Autodesk Inventor part; units mm, degrees
ref_plane "Work Plane2" through (1.7064, 6, 5.9284) normal (0, 0, -1) x (-1, 0, 0)
ref_plane "YZ Plane" through (0, 0, 0) normal (1, 0, 0) x (0, 1, 0)
ref_plane "XZ Plane" through (0, 0, 0) normal (0, 1, 0) x (-1, 0, 0)
sketch "Sketch7" plane through (0, 0, 0) normal (0, 1, 0) x (-1, 0, 0)
  line L0 (-3.4641, -6) -> (-6.9282, 0)
  line L1 (-6.9282, 0) -> (-3.4641, 6)
  line L2 (-3.4641, 6) -> (3.4641, 6)
  line L3 (3.4641, 6) -> (6.9282, 0)
  line L4 (6.9282, 0) -> (3.4641, -6)
  line L5 (3.4641, -6) -> (-3.4641, -6)
  point P0 (0, 0)
  point P1 (0, 0)
  point P2 (0, -6)
  dimension "d24" = 12
extrude "Extrusion6" add sketch "Sketch7" along normal blind 6
sketch "Sketch8" plane through (0, 6, 0) normal (0, 1, 0) x (1, 0, 0)
  circle A0 centre (0, 0) radius 5.5
  circle A1 centre (0, 0) radius 2.575
  line L0 (-0.1332, 2.5716) -> (-0.1332, -1.9284)
  line L1 (-0.1332, -1.9284) -> (-1.7064, -1.9284)
  line L2 (-0.1332, -1.9284) -> (1.7064, -1.9284)
  dimension "d27" = 11
  dimension "d28" = 5.15
  dimension "d29" = 4.5
  dimension "d30" = 1.5732
extrude "Extrusion7" add sketch "Sketch8" along normal blind 18 contours A0 | A1 L1 L2
sketch "Sketch9" plane through (0, 0, 0) normal (0, 0, 1) x (1, 0, 0)
  line L0 (6.9282, 0) -> (3.4641, 0)
  line L1 (6.9282, 0) -> (6.4282, 0)
  line L2 (6.8032, 0.3147) -> (6.4282, 0)
  line L3 (6.9282, 0) -> (6.9282, 0.3868)
  line L4 (0, -4.8) -> (0, 28.8)
  line L5 (6.8032, 0.3147) -> (6.9282, 0.4195)
  line L6 (6.9282, 0.4195) -> (6.9282, 0.3868)
  point P0 (0, 0)
  dimension "d33" = 0.5
  dimension "d35" = 40
  dimension "d39" = 0.125
  dimension "d40" = 0.1049
revolve "Revolution1" cut sketch "Sketch9" angle 360 about axis through (0, -10, 0) along (0, 1, 0)
chamfer "Chamfer3" distance 1 angle 45 2 edges at (0, 24, -2.575) (0, 24, 1.9284)
sketch "Sketch10" plane through (0, 0, 0) normal (0, -1, 0) x (1, 0, 0)
  circle A0 centre (0, 0) radius 1.8
  dimension "d44" = 3.6
extrude "Extrusion8" cut sketch "Sketch10" against normal through all
sketch "Sketch13" plane through (1.7064, 6, 1.9284) normal (0, 0, -1) x (-1, 0, 0)
  circle A0 centre (1.7064, 12) radius 1.8
  point P0 (1.7064, -6)
  dimension "d55" = 3.6
  dimension "d56" = 18
  dimension "d57" = 0
extrude "Extrusion11" cut sketch "Sketch13" against normal through all
ref_plane "Work Plane2" through (1.7064, 6, 5.9284) normal (0, 0, -1) x (-1, 0, 0)
sketch "Sketch14" plane through (1.7064, 6, 5.9284) normal (0, 0, -1) x (-1, 0, 0)
  spline S0 degree 8 poles (3.5064, 12) (3.5064, 12.1901) (3.4834, 12.3798) (3.4377, 12.5672) (3.3691, 12.7503) (3.2769, 12.9271) (3.1607, 13.0947) (3.0198, 13.2496) (2.7182, 13.499) (2.5613, 13.6034) (2.3851, 13.6923) (2.1931, 13.7603) (1.99, 13.8033) (1.7813, 13.819) (1.5725, 13.8069) (1.1492, 13.7262) (0.9448, 13.6548) (0.7585, 13.5594) (0.5918, 13.4445) (0.4454, 13.3144) (0.3197, 13.1725) (0.2144, 13.0225) (0.0308, 12.6885) (-0.0422, 12.5008) (-0.0906, 12.3073) (-0.1146, 12.1105) (-0.1143, 11.9127) (-0.0899, 11.7163) (-0.041, 11.5236) (0.0949, 11.1805) (0.1748, 11.0279) (0.2727, 10.8814) (0.3891, 10.7428) (0.5244, 10.6146) (0.6789, 10.4998) (0.8523, 10.4022) (1.2226, 10.2556) (1.417, 10.2039) (1.6217, 10.1768) (1.8302, 10.1772) (2.0358, 10.2054) (2.2319, 10.2593) (2.4126, 10.3342) (2.8114, 10.5534) (3.0139, 10.7181) (3.1802, 10.9062) (3.3115, 11.1105) (3.409, 11.3257) (3.4738, 11.5476) (3.5064, 11.7733) (3.5064, 12) knots 0 0 0 0 0 0 0 0 0 0.152782 0.152782 0.152782 0.152782 0.152782 0.152782 0.152782 0.27746 0.27746 0.27746 0.27746 0.27746 0.27746 0.27746 0.412202 0.412202 0.412202 0.412202 0.412202 0.412202 0.412202 0.567191 0.567191 0.567191 0.567191 0.567191 0.567191 0.567191 0.697775 0.697775 0.697775 0.697775 0.697775 0.697775 0.697775 0.819734 0.819734 0.819734 0.819734 0.819734 0.819734 0.819734 1 1 1 1 1 1 1 1 1
  circle A0 centre (1.7064, 12) radius 2.5
  line L0 (4.0133, -6) -> (-0.6005, -6)
  point P0 (1.7064, -6)
  point P1 (1.7064, -6)
  point P2 (1.7064, -6)
  dimension "d61" = 5
  dimension "d62" = 18
extrude "Extrusion12" add sketch "Sketch14" along normal up to surface
properties part number "PIN_3DPrint"
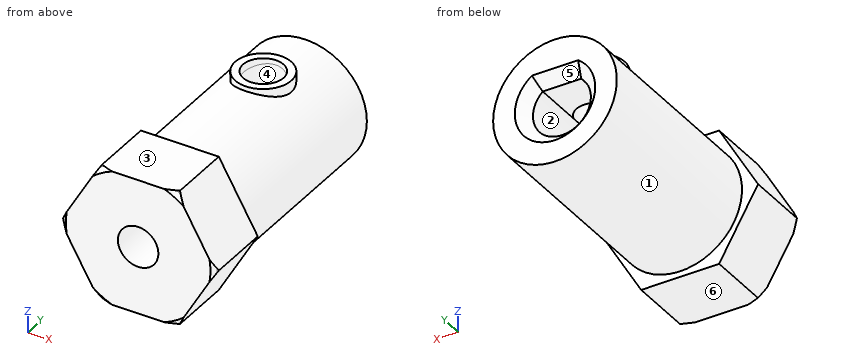
Geometry: final body of the model. Coordinates: model frame, mm. Face numbers are marked on the shaded views. A direction names the side the tool comes from. Coordinates: 2 decimals unless noted, no trailing zeros. Loops run counter-clockwise (first coordinate to the right, second up) from the corner with the lowest first, then second, coordinate; pieces in that order, holes last. Notation, with made-up numbers: M 35.5,53 L 65.5,53 A19 cw 65.5,73 Z; hole C 9.5,1.5 d8. An arc over 180 degrees is marked long. One line per item, written item: value. Start each with the question number.
1) Cut plane D-D (x = 0). Count the separate pieces of the cut face and the enclosed holes in it, then the cut area to 3 significant figures.
2) Pin query (flat end, axial travel): P1, Ø3, axis at x = 0, y = 18, coming from the +Z side; P2, Ø1.7, axis at x = 0, y = 20.5, coming from the -Z side; P3, Ø2, axis at x = 5, y = 18, coming from the +Z side; P4, Ø6.5, axis at x = 0, z = 0, coming from the +Y side. Return the tip coordinate at first contact, or that it passes through.
3) Cut plane B-B (z = 4.5). Return loops of the section in (x, y), then the cut area to 3 significant figures.
4) Cut plane A-A (y = 4). Return loops of the section in (x, z), then the cut area to 3 significant figures.
5) Reachability of the marked faces 4, 5 and 6 from +Z, -Z, +X, -X, +Y, -Y: full face, straight path, thin tool, end or side. Return the list, or none.
6) Draft query along X for the marked faces 1, 2 and 3. Return one class per face: released by +X, released by -X, zero draft, split by the parting line, or undercut.
7) Material intervals for L1, parallel to Y at x = 0, z = 3.3; L2, parallel to X at y = 15.75, z = 0 (3 decimals); L3, parallel to Y at x = -4, z = -5, sorted ascending. Write a range as from..to.
8) Cut plane C-C (x = -5). Return loops of the section in (y, z), then the cut area to 3 significant figures.
Evaluation:
1. separate pieces: 3
1. enclosed holes: 0
1. area: 154 mm^2
2. P1: z = -2.09
2. P2: z = -5.5
2. P3: z = 3.77
2. P4: y = 24
3. outline: M -4.33,0 L 4.33,0 L 4.33,6 L 3.16,6 L 3.16,24 L -3.16,24 L -3.16,6 L -4.33,6 Z; hole C 0,18 d3.6
3. area: 156 mm^2
4. outline: M -6.93,0 L -3.46,-6 L 3.46,-6 L 6.93,0 L 3.46,6 L -3.46,6 Z; hole C 0,0 d3.6
4. area: 115 mm^2
5. face 4: +Z
5. face 5: +Y
5. face 6: -Z, +X, -X, +Y, -Y
6. face 1: split by the parting line
6. face 2: undercut
6. face 3: zero draft
7. L1: 0..16.2, 19.8..24
7. L2: -5.5..-2.575, 2.575..5.5
7. L3: 0..6
8. outline: M 0,-3.34 L 6,-3.34 L 6,-2.29 L 24,-2.29 L 24,2.29 L 6,2.29 L 6,3.34 L 0,3.34 Z
8. area: 123 mm^2
